Part print with two shaded views. Sizes in mm from the minimum x, y, z corner. A direction names the side the tool comes from. Round coordinates to 2 decimals unless told otherwise and drop trailing zeros. Order: outer loops, then holes, each group sorted by start corner. A loop starts at its lowest first (then second) coordinate and runs counter-clockwise, first axis right, second up. Notation, with made-up numbers: M 11,32.5 L 38,32.5 A33 ccw 38,69.5 Z; hole C 80.25,35 d9. An arc over 180 degrees is marked long. Return JSON: item names as keys, results as strings. Group by question number.
Item 1: Pin check, flat tips, straight feed: pin 1 Ø7.5 at (x, z) = (20, 36) entering from -Y; pin 2 Ø12 at (x, y) = (87, 36.5) entering from -Z. Stop position of each tip, or through.
Item 2: Probe line 1 along Z through (x, y) = (80, 53.3); line 2 along X through (y, z) = (43.5, 10.5); line 3 along X through (y, z) = (54, 36). List the from-to ranges inside material, lowest first.
Item 3: Which spindle directions (+Z, -Z, +X, -X, +Y, -Y) get a long thin tool onto all of the face, cutting with end or side? Do the marked faces 4 and 5. Say none if no direction does.
Item 4: Slice it at B-B on z = 36. Write the cut outline in (x, y), then the cut area to 3 significant figures.
Item 5: Slice it at C-C on x = 80. Write the cut outline in (y, z), then the cut area to 3 significant figures.
Item 6: Slice it at A-A on y = 31. Write the cut outline in (x, z), then the cut area to 3 significant figures.
Item 7: Slice it at D-D on z = 5.5. Write the cut outline in (x, y).
Item 8: Pull direction X, two halves, no side cores. Call the marked faces 1, 2 and 3: pulls with the +X half, pulls with the -X half, needs draft (parallel to the pull), parting line crosses it, or undercut.
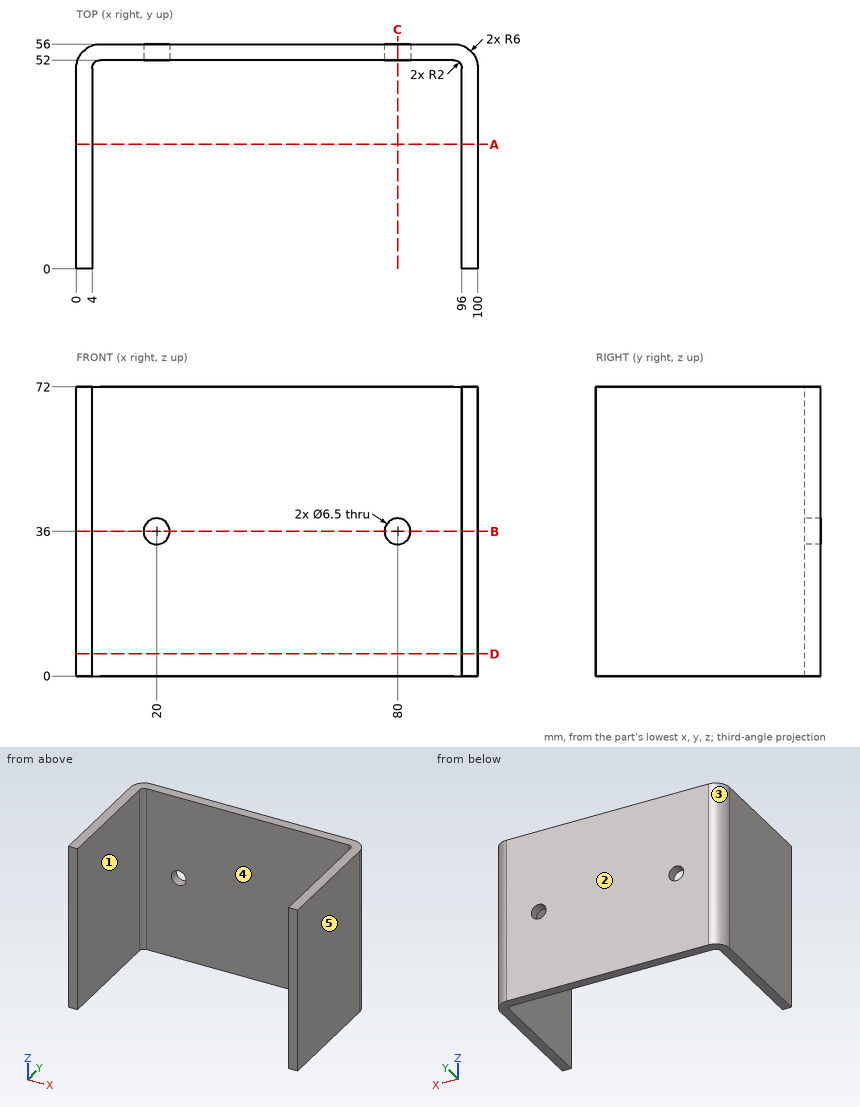
Output values:
{
 "1": {"pin 1": "y = 52", "pin 2": "through"},
 "2": {"line 1": "0 to 32.75, 39.25 to 72", "line 2": "0 to 4, 96 to 100", "line 3": "1.53 to 16.75, 23.25 to 76.75, 83.25 to 98.47"},
 "3": {"face 4": "+Z, -Z, -Y", "face 5": "+Z, -Z, +X, +Y, -Y"},
 "4": {"outline": "M 0,0 L 4,0 L 4,50 A2 cw 6,52 L 16.75,52 L 16.75,56 L 6,56 A6 ccw 0,50 Z; M 23.25,52 L 76.75,52 L 76.75,56 L 23.25,56 Z; M 83.25,52 L 94,52 A2 cw 96,50 L 96,0 L 100,0 L 100,50 A6 ccw 94,56 L 83.25,56 Z", "area": "750 mm²"},
 "5": {"outline": "M 52,0 L 56,0 L 56,32.75 L 52,32.75 Z; M 52,39.25 L 56,39.25 L 56,72 L 52,72 Z", "area": "262 mm²"},
 "6": {"outline": "M 0,0 L 4,0 L 4,72 L 0,72 Z; M 96,0 L 100,0 L 100,72 L 96,72 Z", "area": "576 mm²"},
 "7": {"outline": "M 0,0 L 4,0 L 4,50 A2 cw 6,52 L 94,52 A2 cw 96,50 L 96,0 L 100,0 L 100,50 A6 ccw 94,56 L 6,56 A6 ccw 0,50 Z"},
 "8": {"face 1": "undercut", "face 2": "needs draft", "face 3": "pulls with the -X half"}
}
